Input: part model. Units: mm. Frame: model coordinates. A direction names the side the tool comes from. Coordinates: 2 decimals unless noted, no trailing zeros. Loops run counter-clockwise (first coordinate to the right, second up) from the corner with the lowest first, then second, coordinate; pieces in that order, holes last.
(1) Set-up query: faces 1 (the face through (-5.75, 74, 27)), 2 (the face through (18.25, 55, 18)), 3 (the face through (8, 24, 17)), 4 (the face through (7.35, -0.95, -22.15)), 5 (the face through (26.25, 55, 16)). Return all of +Z, -Z, +X, -X, +Y, -Y with unobstructed straight access to the full face (end or side cutting, diameter ignored); none if empty.
(2) Section B-B, the plane y = 45. Return loops of the section in (x, z), then the cut area to 3 significant figures.
(3) Section D-D, the plane y = 27.5. Return loops of the section in (x, z), then the cut area to 4 significant figures.
(4) Section A-A, the plane z = -30. Return loops of the section in (x, y), then the cut area to 3 significant figures.
(5) Section C-C, the plane x = 11.5. Return loops of the section in (y, z).
(6) Mould query, pull axis Y, two halves, no side actions, for faces 6 (the face through (23.292, 75.415, 25.894)), 7 (the face through (7.352, -29.745, -43.351)), 8 (the face through (16.35, 33.1, 8.62)). Classes: released by +Y, released by -Y, zero draft, split by the parting line, or undercut.
(7) Contact query for flat-ended pins moving along their axis: P1, Ø20, axis at y = -21.46, z = -32.06, coming from the +X side; P2, Ø2, axis at x = 14.5, y = -1, coming from the +Z side; P3, Ø11.5, axis at x = -0.5, y = 35.5, coming from the -Z side; P4, Ø12, axis at x = 9.5, z = 4.5, coming from the -Y side. Output: stop coordinate, or through.
(8) Line query: L1, parallel to X at y = 71, z = 37; L2, parallel to X at y = 42, z = 12.5; L3, parallel to Z at x = 3, y = -27. Output: solid intervals per line, ascending.
```python
from build123d import *

# Parameters (mm, degrees)
EXTRUDE_1_DEPTH      = 23
CUT_EXTRUDE_1_DEPTH  = 70.412264766
EXTRUDE_7_REACH      = 76.653
EXTRUDE_8_DEPTH      = 38
SKETCH_18_R          = 7.5
CUT_EXTRUDE_10_DEPTH = 97.091099475
SKETCH_16_W          = 22
SKETCH_16_H          = 105.274199252
CUT_EXTRUDE_9_DEPTH  = 60.342228518
EXTRUDE_5_DEPTH      = 14.5
EXTRUDE_6_DEPTH      = 14.5
SKETCH_14_R          = 11
CUT_EXTRUDE_8_DEPTH  = 14.5
SKETCH_19_R          = 9.5
CUT_EXTRUDE_11_DEPTH = 6
CUT_EXTRUDE_START    = -6
SKETCH_20_R          = 9.5
CUT_EXTRUDE_12_DEPTH = 6
CUT_EXTRUDE_13_DEPTH = 42
CUT_EXTRUDE_14_DEPTH = 42
FILLET_1_R           = 10


with BuildPart() as part:
    # 草图1 → 凸台-拉伸1 (new body)
    with BuildSketch(Plane.XY):
        Polygon((0, 0), (14.5, 0), (14.5, 20), (26.25, 31.75), (26.25, 60), (18.25, 60), (18.25, 35), (-3.75, 35), (-3.75, 60), (-11.75, 60), (-11.75, 31.75), (0, 20), align=None)
    extrude(amount=EXTRUDE_1_DEPTH)

    # 草图2 → 切除-拉伸1 (cut, through all)
    with BuildSketch(Plane.XY.offset(23)):
        Polygon((-3.75, 35), (0, 31.25), (14.5, 31.25), (18.25, 35), align=None)
    extrude(amount=-CUT_EXTRUDE_1_DEPTH, mode=Mode.SUBTRACT)

    # 凸台-拉伸7: up to this face of the body (flat: up to its plane)
    extrude_7_end = Plane(part.part.faces().sort_by_distance((-11.75, 45.875, 11.5))[0])
    # 草图15 → 凸台-拉伸7 (add, up to the picked face)
    with BuildSketch(Plane(origin=(26.25, 0, 0), x_dir=(0, 0, -1), z_dir=(1, 0, 0)), mode=Mode.PRIVATE) as extrude_7_sk1:
        Polygon((0, 60), (-22.93625724, 76.060140218), (-36.128515276, 57.219643199), (-23, 48.026957837), align=None)
    extrude_7_tool1 = split(extrude(extrude_7_sk1.sketch, amount=-EXTRUDE_7_REACH, mode=Mode.PRIVATE), bisect_by=extrude_7_end, keep=Keep.BOTH, mode=Mode.PRIVATE)
    add(extrude_7_tool1.solids().sort_by(Axis((26.25, 61.024992, 19.695992), (-1, 0, 0)))[0])

    # 草图17 → 凸台-拉伸8 (add)
    with BuildSketch(Plane(origin=(26.25, 0, 0), x_dir=(0, 0, -1), z_dir=(1, 0, 0))):
        with BuildLine():
            Line((-22.93625724, 76.060140218), (-36.128515276, 57.219643199))
            ThreePointArc((-36.128515276, 57.219643199), (-38.952634767, 73.236020727), (-22.93625724, 76.060140218))
        make_face()
    extrude(amount=-EXTRUDE_8_DEPTH)

    # 草图18 → 切除-拉伸10 (cut, through all)
    with BuildSketch(Plane(origin=(26.25, 0, 0), x_dir=(0, 0, -1), z_dir=(1, 0, 0))):
        with Locations(Location((-29.532386258, 66.639891709, 0), (0, 0, 90))):
            Circle(SKETCH_18_R)
    extrude(amount=-CUT_EXTRUDE_10_DEPTH, mode=Mode.SUBTRACT)

    # 草图16 → 切除-拉伸9 (cut, through all)
    with BuildSketch(Plane(origin=(0, 47.207293091, 24.574561329), x_dir=(1, 0, 0), z_dir=(0, -0.8870108331782229, -0.4617486132350318))):
        with Locations((7.25, 24.932182832)):
            Rectangle(SKETCH_16_W, SKETCH_16_H)
    extrude(amount=-CUT_EXTRUDE_9_DEPTH, mode=Mode.SUBTRACT)

    # 草图12 → 凸台-拉伸5 (add)
    with BuildSketch(Plane(origin=(14.5, 0, 0), x_dir=(0, 0, -1), z_dir=(1, 0, 0))):
        Polygon((0, 18.076915106), (40.09243026, -9.996106787), (24.032290042, -32.932364027), (-23, 0), align=None)
    extrude(amount=-EXTRUDE_5_DEPTH)

    # 草图13 → 凸台-拉伸6 (add)
    with BuildSketch(Plane(origin=(14.5, 0, 0), x_dir=(0, 0, -1), z_dir=(1, 0, 0))):
        with BuildLine():
            Line((40.09243026, -9.996106787), (24.032290042, -32.932364027))
            ThreePointArc((24.032290042, -32.932364027), (43.530488771, -29.494305516), (40.09243026, -9.996106787))
        make_face()
    extrude(amount=-EXTRUDE_6_DEPTH)

    # 草图14 → 切除-拉伸8 (cut)
    with BuildSketch(Plane(origin=(14.5, 0, 0), x_dir=(0, 0, -1), z_dir=(1, 0, 0))):
        with Locations((32.062360151, -21.464235407)):
            Circle(SKETCH_14_R)
    extrude(amount=-CUT_EXTRUDE_8_DEPTH, mode=Mode.SUBTRACT)

    # 草图19 → 切除-拉伸11 (cut)
    with BuildSketch(Plane(origin=(26.25, 0, 0), x_dir=(0, 0, -1), z_dir=(1, 0, 0))):
        with Locations(Location((-29.532386258, 66.639891709, 0), (0, 0, 90))):
            Circle(SKETCH_19_R)
    extrude(amount=-CUT_EXTRUDE_11_DEPTH, mode=Mode.SUBTRACT)

    # 草图20 → 切除-拉伸12 (cut)
    with BuildSketch(Plane.ZY.offset(11.75).offset(CUT_EXTRUDE_START)):
        with Locations(Location((29.532386258, 66.639891709, 0), (0, 0, 90))):
            Circle(SKETCH_20_R)
    extrude(amount=CUT_EXTRUDE_12_DEPTH, mode=Mode.SUBTRACT)

    # 草图21 → 切除-拉伸13 (cut)
    with BuildSketch(Plane(origin=(26.25, 0, 0), x_dir=(0, 0, -1), z_dir=(1, 0, 0))):
        Polygon((-23, 48.026957837), (-17, 43.825712608), (-17, -13.167272348), (-41.854258514, 0), align=None)
    extrude(amount=-CUT_EXTRUDE_13_DEPTH, mode=Mode.SUBTRACT)

    # 草图22 → 切除-拉伸14 (cut)
    with BuildSketch(Plane(origin=(14.5, 0, 0), x_dir=(0, 0, -1), z_dir=(1, 0, 0))):
        with BuildLine():
            Line((0, 18.076915106), (0, 10))
            Line((0, 10), (39.195351346, -9.373093948))
            ThreePointArc((39.195351346, -9.373093948), (42.389326913, -11.954817829), (44.699464232, -15.350409632))
            Line((44.699464232, -15.350409632), (51.638294373, -1.311873193))
            Line((51.638294373, -1.311873193), (0, 18.076915106))
        make_face()
    extrude(amount=-CUT_EXTRUDE_14_DEPTH, mode=Mode.SUBTRACT)

    # 圆角1
    fillet_1_edges = [part.edges().sort_by_distance(p)[0] for p in [
        (-7.75, 60, 0),
        (22.25, 60, 0),
        (7.25, -4.201245229, 17),
        (22.25, 43.825712608, 17),
        (-7.75, 43.825712608, 17),
        (7.25, 10, 0),
    ]]
    fillet(fillet_1_edges, radius=FILLET_1_R)


solid = part.part
```
Report:
1. face 1: -X
1. face 2: +Z, -Z, +Y
1. face 3: +Z, +X, -X, -Y
1. face 4: -Z, +X, -X, +Y
1. face 5: +Z, -Z, +X, +Y, -Y
2. outline: (-11.75, 0) - (-3.75, 0) - (-3.75, 19.3) - (-11.75, 19.3) - close; (18.25, 0) - (26.25, 0) - (26.25, 19.3) - (18.25, 19.3) - close
2. area: 309 mm2
3. outline: (-7.5, 0) - (22, 0) - (22, 17) - (-7.5, 17) - close
3. area: 501.5 mm2
4. outline: (0, -35.31) - (14.5, -35.31) - (14.5, -32.27) - (0, -32.27) - close; (0, -10.66) - (14.5, -10.66) - (14.5, -4.83) - (0, -4.83) - close
4. area: 129 mm2
5. outline: (-32.93, -24.03) arc R14 ccw to (-10, -40.09) - (-9.4, -39.24) arc R14.04 ccw to (-9.37, -39.2) - (7.25, -5.57) arc R10 cw to (16.21, 0) - (31.25, 0) - (31.25, 17) - (1, 17) arc R10 ccw to (-7.19, 12.74) - close; hole circle Ø22 at (-21.46, -32.06)
6. face 6: undercut
6. face 7: split by the parting line
6. face 8: released by +Y
7. P1: passes through
7. P2: stops at z = 16.95
7. P3: stops at z = 0
7. P4: stops at y = -17.16
8. L1: x = -5.75 to -3.75, 18.25 to 20.25
8. L2: x = -11.75 to -3.75, 18.25 to 26.25
8. L3: z = -44.92 to -41.57, -22.56 to -15.56
